from build123d import *

# Parameters (mm, degrees)
BOSS_EXTRUDE1_DEPTH = 1.5
SKETCH2_W           = 0.55
SKETCH2_H           = 0.548166652
BOSS_EXTRUDE2_DEPTH = 8.3


with BuildPart() as part:
    # Sketch1 → Boss-Extrude1 (new body)
    with BuildSketch(Plane.XY):
        Polygon((-1.929641956, 0), (2.070358044, 0), (2.570358044, 0.504083326), (2.570358044, 2.044083326), (2.066274717, 2.544083326), (-1.933725283, 2.544083326), (-2.433725283, 2.04), (-2.433725283, 0.5), align=None)
    extrude(amount=BOSS_EXTRUDE1_DEPTH)

    # Sketch2 → Boss-Extrude2 (add)
    with BuildSketch(Plane.XY.offset(1.5)):
        with Locations((-1.198725283, 1.27)):
            Rectangle(SKETCH2_W, SKETCH2_H)
        Polygon((1.611236473, 1.000868125), (1.061239307, 0.999102598), (1.059479665, 1.547266427), (1.609476832, 1.549031954), align=None)
    extrude(amount=BOSS_EXTRUDE2_DEPTH)


solid = part.part
The model under review builds one solid part; all positions refer to its coordinate system, in mm. Give positions to 0.01 mm unless a question says otherwise; leave off trailing zeros. Loops run counter-clockwise (first coordinate to the right, second up) from the corner with the lowest first, then second, coordinate; pieces in that order, holes last. Notation, with made-up numbers: (78, 33) -> (96, 33) arc R25 cw to (96, 52) -> close; hole circle Ø2 at (-24, 64.25). An arc over 180 degrees is marked (long way). Put each result on its own line as item: value. Start each with the question number.
1. Wall thickness on probe 1 along X at (y, z) = (1.25, 7.75); probe 2 along Z at (x, y) = (-1.95, 0.95); probe 3 along Y at (x, z) = (-1.25, 4.5): over which ranges is each line inside the solid? List them lowest first.
2. We need section C-C on x = 0.6. State the section outline as (y, z) points, then the cut area to 3 significant figures.
3. Clearance check with a flat-ended pin moving along its axis: P1, Ø0.6, axis at x = -1, z = 5, coming from the -Y side. State where the tip first meets the part, or that it passes through.
4. We need section D-D on x = 1.5. State the section outline as (y, z) points, then the cut area to 3 significant figures.
5. We need section A-A on z = 9. State the section outline as (x, y) points, then the cut area to 3 significant figures.
6. We need section B-B on y = 1.3. State the section outline as (x, z) points.
Determined:
1. probe 1: -1.47 to -0.92, 1.06 to 1.61
1. probe 2: 0 to 1.5
1. probe 3: 1 to 1.54
2. outline: (0, 0) -> (2.54, 0) -> (2.54, 1.5) -> (0, 1.5) -> close
2. area: 3.82 mm^2
3. P1: y = 1
4. outline: (0, 0) -> (2.54, 0) -> (2.54, 1.5) -> (1.55, 1.5) -> (1.55, 9.8) -> (1, 9.8) -> (1, 1.5) -> (0, 1.5) -> close
4. area: 8.37 mm^2
5. outline: (-1.47, 1) -> (-0.92, 1) -> (-0.92, 1.54) -> (-1.47, 1.54) -> close; (1.06, 1) -> (1.61, 1) -> (1.61, 1.55) -> (1.06, 1.55) -> close
5. area: 0.603 mm^2
6. outline: (-2.43, 0) -> (2.57, 0) -> (2.57, 1.5) -> (1.61, 1.5) -> (1.61, 9.8) -> (1.06, 9.8) -> (1.06, 1.5) -> (-0.92, 1.5) -> (-0.92, 9.8) -> (-1.47, 9.8) -> (-1.47, 1.5) -> (-2.43, 1.5) -> close
